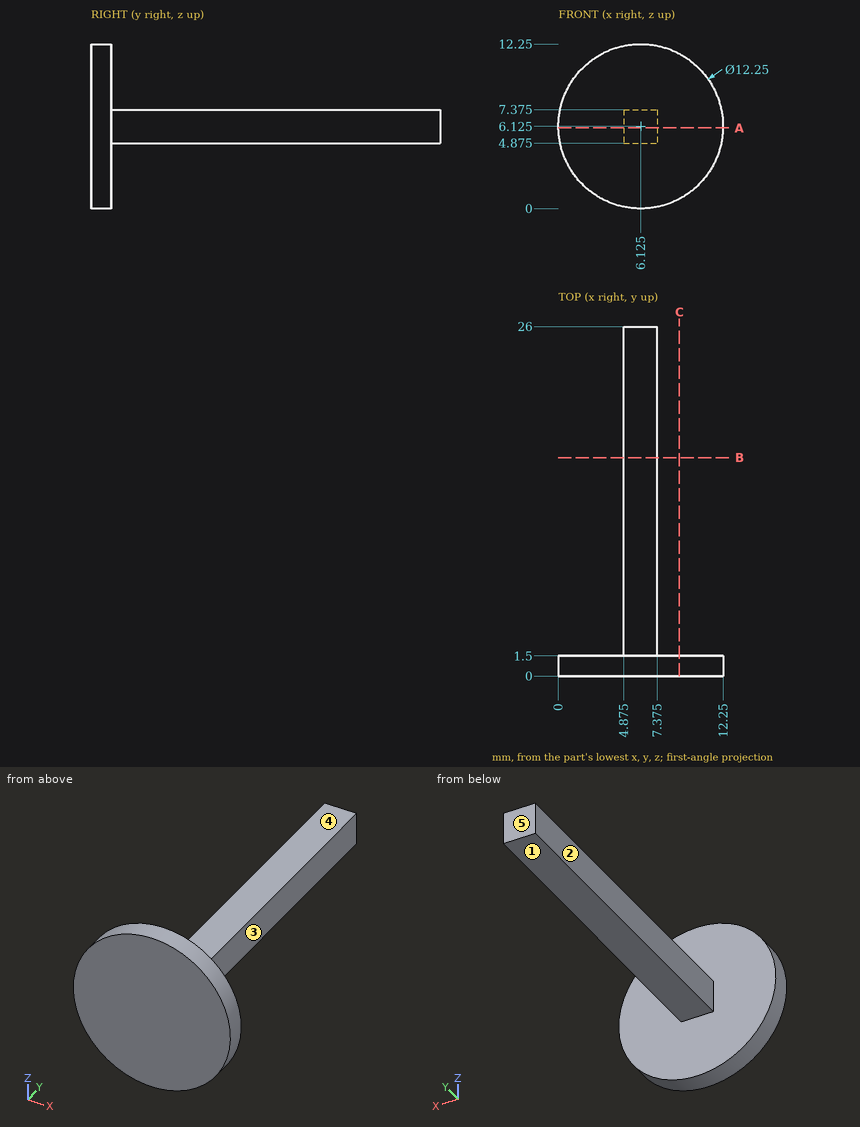
The figure shows three views and two pictorial views of one solid part (mm, origin at its lowest corner). Answer the questions. A direction names the side the tool comes from. Coordinates: 2 decimals unless noted, no trailing zeros. Order: outer loops, then holes, each group sorted by start corner. A loop starts at its lowest first (then second) coordinate and runs counter-clockwise, first axis right, second up. Notation, with made-up numbers: (19, 68) - (62, 68) arc R20 cw to (62, 91) - close; hole circle Ø10 at (60.5, -16.5). An arc over 180 degrees is marked (long way). Answer as a JSON object with one key per item and string values.
1. Consider line 1 (Y direction, x = 6.5, z = 1.5); line 2 (X direction, y = 9.25, z = 6.5) (3 decimals). Determine where each line is inside the solid, lowest interval first.
Output values:
{"line 1": "y = 0 to 1.5", "line 2": "x = 4.875 to 7.375"}
2. A tool of negligible diameter and unlimited length cuts with its end or side. For the marked faces 1, 2, 3, 4 and 5, from which of +Z, -Z, +X, -X, +Y, -Y can it reach the whole face along a straight path? Write none if from no direction.
Output values:
{"face 1": "-Z, +X, -X, +Y", "face 2": "+Z, -Z, -X, +Y", "face 3": "+Z, -Z, +X, +Y", "face 4": "+Z, +X, -X, +Y", "face 5": "+Z, -Z, +X, -X, +Y"}
3. Find section B-B on y = 16.25. Determine the outline of the cut face in (x, z) (3 decimals), plus the area to 3 significant figures.
Output values:
{"outline": "(4.875, 4.875) - (7.375, 4.875) - (7.375, 7.375) - (4.875, 7.375) - close", "area": "6.25 mm²"}
4. Find section C-C on x = 9. Determine the outline of the cut face in (y, z), plus the area to 3 significant figures.
Output values:
{"outline": "(0, 0.72) - (1.5, 0.72) - (1.5, 11.53) - (0, 11.53) - close", "area": "16.2 mm²"}
5. Each of these flat-tipped pins is pushed along its axis until it touches: P1, Ø0.8, axis at x = 6, y = 9, coming from the +Z side (3 decimals); P2, Ø2, axis at x = 6, y = 14, coming from the -Z side (3 decimals); P3, Ø1.2, axis at y = 10, z = 6.5, coming from the +X side (3 decimals). Where does it stop, or does it pass through?
Output values:
{"P1": "stops at z = 7.375", "P2": "stops at z = 4.875", "P3": "stops at x = 7.375"}
6. Find section A-A on z = 6. Determine the outline of the cut face in (x, y) (3 decimals), plus the area to 3 significant figures.
Output values:
{"outline": "(0.001, 0) - (12.249, 0) - (12.249, 1.5) - (7.375, 1.5) - (7.375, 26) - (4.875, 26) - (4.875, 1.5) - (0.001, 1.5) - close", "area": "79.6 mm²"}
